Geometry check sheet. Reference: the model listing, model coordinates, mm. Face numbers are marked on the shaded views. A direction names the side the tool comes from. Coordinates: 2 decimals unless noted, no trailing zeros. Loops run counter-clockwise (first coordinate to the right, second up) from the corner with the lowest first, then second, coordinate; pieces in that order, holes last. Notation, with made-up numbers: M 26,11 L 67,11 A12 ccw 67,18 Z; hole C 1,-7 d6. An arc over 180 degrees is marked long. One line per question, with ' | ' between items. Start each with the question number.
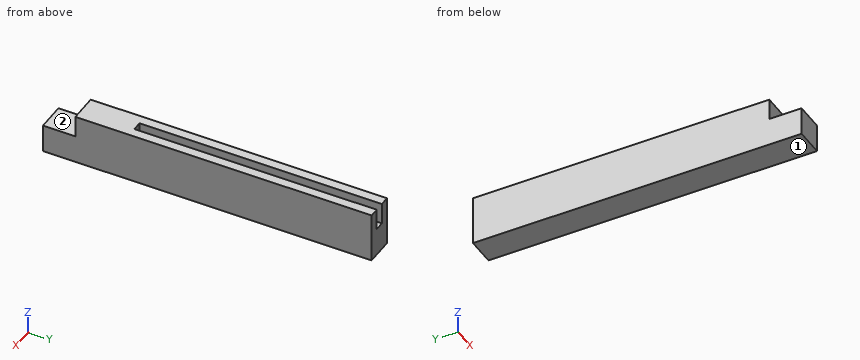
from build123d import *

# Parameters (mm, degrees)
SKETCH1_W           = 5.25
SKETCH1_H           = 5.25
BOSS_EXTRUDE1_DEPTH = 6
SKETCH2_W           = 5.25
SKETCH2_H           = 9.25
BOSS_EXTRUDE2_DEPTH = 55
SKETCH3_W           = 1.75
SKETCH3_H           = 8
CUT_EXTRUDE1_DEPTH  = 45


with BuildPart() as part:
    # Sketch1 → Boss-Extrude1 (new body)
    with BuildSketch(Plane(origin=(0, 0, 0), x_dir=(1, 0, 0), z_dir=(0, 1, 0))):
        Rectangle(SKETCH1_W, SKETCH1_H)
    extrude(amount=BOSS_EXTRUDE1_DEPTH)

    # Sketch2 → Boss-Extrude2 (add)
    with BuildSketch(Plane(origin=(0, 6, 0), x_dir=(1, 0, 0), z_dir=(0, 1, 0))):
        with Locations((0, -2)):
            Rectangle(SKETCH2_W, SKETCH2_H)
    extrude(amount=BOSS_EXTRUDE2_DEPTH)

    # Sketch3 → Cut-Extrude1 (cut)
    with BuildSketch(Plane(origin=(0, 61, 0), x_dir=(1, 0, 0), z_dir=(0, 1, 0))):
        with Locations((0, -6.625)):
            Rectangle(SKETCH3_W, SKETCH3_H)
    extrude(amount=-CUT_EXTRUDE1_DEPTH, mode=Mode.SUBTRACT)


solid = part.part
1. Tool access check on the marked faces 1 and 2. Record the directions out of +Z, -Z, +X, -X, +Y, -Y that give a thin tool (end or side, any length) a straight path to the whole face; none if there is none.
2. Depth check by flat-ended pin: pin 1 Ø1.6 at (x, y) = (-0.5, 2.5) entering from +Z (3 decimals). Enter the tip coordinate at first touch or a pass-through.
3. Sectioned sample at B-B (y = 54). Record the cut outline in (x, z) (3 decimals), and give its area (3 significant figures).
4. Sectioned sample at A-A (x = 0.35). Record the cut outline in (y, z) (3 decimals), and give its area (3 significant figures).
5. Thickness scan on line 1 (X direction, y = 23, z = 6) (3 decimals); line 2 (Z direction, x = 0.75, y = 38) (3 decimals); line 3 (Y direction, x = -2.25, z = 6). Record the ranges inside material, lowest first.
Result:
1) face 1: -Z, +X, -X, +Y, -Y | face 2: +Z, +X, -X, -Y
2) pin 1: stops at z = 2.625
3) outline: M -2.625,-2.625 L 2.625,-2.625 L 2.625,6.625 L 0.875,6.625 L 0.875,2.625 L -0.875,2.625 L -0.875,6.625 L -2.625,6.625 Z | area: 41.6 mm2
4) outline: M 0,-2.625 L 61,-2.625 L 61,2.625 L 16,2.625 L 16,6.625 L 6,6.625 L 6,2.625 L 0,2.625 Z | area: 360 mm2
5) line 1: x = -2.625 to -0.875, 0.875 to 2.625 | line 2: z = -2.625 to 2.625 | line 3: y = 6 to 61
